```python
from build123d import *

# Parameters (mm, degrees)
PAD_DEPTH              = 6.05
SKETCH_W               = 3.6
SKETCH_H               = 14.9
POCKET_DEPTH           = 4.3
POCKET001_DEPTH        = 1.45
POCKET001_DEPTH_BACK   = 13.45
SKETCH004_W            = 0.55
SKETCH004_H            = 10
POCKET002_DEPTH        = 4.3
SKETCH005_W            = 1.2
SKETCH005_H            = 2.2
POCKET003_DEPTH        = 1.751
POCKET004_DEPTH        = 2.001
POCKET004_DEPTH_BACK   = 14.001
SKETCH007_W            = 0.5
SKETCH007_H            = 0.5
POCKET005_DEPTH        = 2.001
POCKET005_DEPTH_BACK   = 14.001
SKETCH008_W            = 0.2
SKETCH008_H            = 0.45
PAD001_DEPTH           = 4.85
LINEARPATTERN_COUNT    = 6
LINEARPATTERN_PITCH    = 2
POCKET006_DEPTH        = 12
SKETCH010_W            = 1.6
SKETCH010_H            = 0.2
POCKET007_DEPTH        = 2.951
POCKET007_DEPTH_BACK   = 1.751
LINEARPATTERN001_COUNT = 7
LINEARPATTERN001_PITCH = 2
SKETCH011_W            = 0.5
SKETCH011_H            = 0.5
POCKET008_DEPTH        = 0.001
POCKET008_DEPTH_BACK   = 6.051
LINEARPATTERN002_COUNT = 7
LINEARPATTERN002_PITCH = 2


with BuildPart() as part:
    # Sketch001 → Pad (new body)
    with BuildSketch(Plane.XY):
        with BuildLine():
            Line((-2.95, 1.5), (-2.95, -13.5))
            ThreePointArc((-2.95, -13.5), (-2.803553, -13.853553), (-2.45, -14))
            Line((-2.45, -14), (1.25, -14))
            ThreePointArc((1.25, -14), (1.603553, -13.853553), (1.75, -13.5))
            Line((1.75, -13.5), (1.75, 1.5))
            ThreePointArc((1.75, 1.5), (1.603553, 1.853553), (1.25, 2))
            Line((1.25, 2), (-2.45, 2))
            ThreePointArc((-2.45, 2), (-2.803553, 1.853553), (-2.95, 1.5))
        make_face()
    extrude(amount=PAD_DEPTH)

    # Sketch (on DatumPlane) → Pocket (cut)
    with BuildSketch(Plane.XY.offset(6.05)):
        with Locations((-0.6, -6)):
            Rectangle(SKETCH_W, SKETCH_H)
    extrude(amount=-POCKET_DEPTH, mode=Mode.SUBTRACT)

    # Sketch003 → Pocket001 (cut, two sides)
    with BuildSketch(Plane.XZ) as pocket001_sk:
        Polygon((1.5, 6.05), (1.2, 6.05), (1.2, 5.55), align=None)
        Polygon((-2.7, 6.05), (-2.4, 5.55), (-2.4, 6.05), align=None)
        Polygon((-2.4, 1.75), (-0.3, 1.75), (-0.9, 1.07), (-2.4, 1.07), align=None)
    extrude(amount=-POCKET001_DEPTH, mode=Mode.SUBTRACT)
    extrude(pocket001_sk.sketch, amount=POCKET001_DEPTH_BACK, mode=Mode.SUBTRACT)

    # Sketch004 (on DatumPlane) → Pocket002 (cut)
    with BuildSketch(Plane.XY.offset(6.05)):
        with Locations((1.475, -6)):
            Rectangle(SKETCH004_W, SKETCH004_H)
    extrude(amount=-POCKET002_DEPTH, mode=Mode.SUBTRACT)

    # Sketch005 → Pocket003 (cut, through all)
    with BuildSketch(Plane.YZ):
        with Locations((0.85, 2.93)):
            Rectangle(SKETCH005_W, SKETCH005_H)
        with Locations((-12.85, 2.93)):
            Rectangle(SKETCH005_W, SKETCH005_H)
    extrude(amount=POCKET003_DEPTH, mode=Mode.SUBTRACT)

    # Sketch006 → Pocket004 (cut, two sides)
    with BuildSketch(Plane.XZ) as pocket004_sk:
        with BuildLine():
            Line((0.45, 5.85), (0.45, 4.05))
            Line((0.45, 4.05), (-0.55, 4.05))
            Line((-0.55, 4.05), (-0.55, 5.85))
            ThreePointArc((-0.55, 5.85), (-0.608579, 5.991421), (-0.75, 6.05))
            Line((0.65, 6.05), (-0.75, 6.05))
            ThreePointArc((0.65, 6.05), (0.508579, 5.991421), (0.45, 5.85))
        make_face()
    extrude(amount=-POCKET004_DEPTH, mode=Mode.SUBTRACT)
    extrude(pocket004_sk.sketch, amount=POCKET004_DEPTH_BACK, mode=Mode.SUBTRACT)

    # Sketch007 → Pocket005 (cut, two sides)
    with BuildSketch(Plane.XZ) as pocket005_sk:
        with Locations((1.5, 0.95)):
            Rectangle(SKETCH007_W, SKETCH007_H)
    extrude(amount=-POCKET005_DEPTH, mode=Mode.SUBTRACT)
    extrude(pocket005_sk.sketch, amount=POCKET005_DEPTH_BACK, mode=Mode.SUBTRACT)

    # Sketch008 → Pad001 (join)
    with BuildSketch(Plane.XY):
        with Locations((-2.3, -1)):
            Rectangle(SKETCH008_W, SKETCH008_H)
    pad001 = extrude(amount=PAD001_DEPTH)

    # LinearPattern: Pad001 ×6
    with Locations(*[(0, -i * LINEARPATTERN_PITCH, 0) for i in range(1, LINEARPATTERN_COUNT)]):
        add(pad001)

    # Sketch009 → Pocket006 (cut)
    with BuildSketch(Plane.XZ):
        with BuildLine():
            Line((-2.4, 4.95), (-2.2, 4.95))
            Line((-2.2, 4.95), (-2.2, 4.65))
            ThreePointArc((-2.2, 4.65), (-2.258579, 4.791421), (-2.4, 4.85))
            Line((-2.4, 4.85), (-2.4, 4.95))
        make_face()
    extrude(amount=POCKET006_DEPTH, mode=Mode.SUBTRACT)

    # Sketch010 → Pocket007 (cut, two sides)
    with BuildSketch(Plane.YZ) as pocket007_sk:
        with Locations((0, 0.1)):
            Rectangle(SKETCH010_W, SKETCH010_H)
    pocket007 = extrude(amount=-POCKET007_DEPTH, mode=Mode.SUBTRACT) + extrude(pocket007_sk.sketch, amount=POCKET007_DEPTH_BACK, mode=Mode.SUBTRACT)

    # LinearPattern001: Pocket007 ×7
    with Locations(*[(0, -i * LINEARPATTERN001_PITCH, 0) for i in range(1, LINEARPATTERN001_COUNT)]):
        add(pocket007, mode=Mode.SUBTRACT)

    # Sketch011 → Pocket008 (cut, two sides)
    with BuildSketch(Plane.XY) as pocket008_sk:
        Rectangle(SKETCH011_W, SKETCH011_H)
    pocket008 = extrude(amount=-POCKET008_DEPTH, mode=Mode.SUBTRACT) + extrude(pocket008_sk.sketch, amount=POCKET008_DEPTH_BACK, mode=Mode.SUBTRACT)

    # LinearPattern002: Pocket008 ×7
    with Locations(*[(0, -i * LINEARPATTERN002_PITCH, 0) for i in range(1, LINEARPATTERN002_COUNT)]):
        add(pocket008, mode=Mode.SUBTRACT)


solid = part.part
```
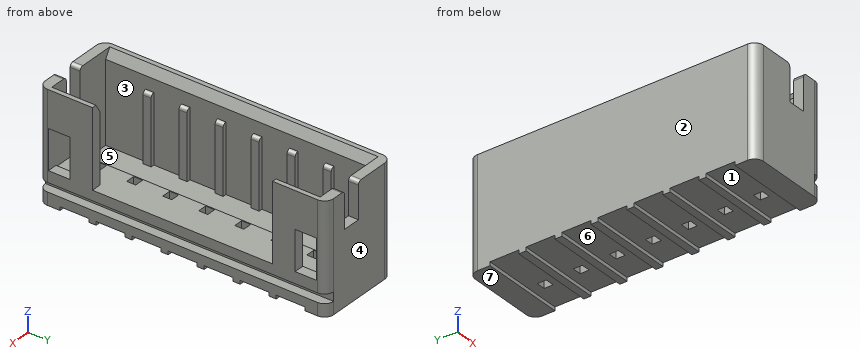
Geometry check sheet. Reference: the model listing, model coordinates, mm. Face numbers are marked on the shaded views. A direction names the side the tool comes from. Coordinates: 2 decimals unless noted, no trailing zeros. Order: outer loops, then holes, each group sorted by start corner. A loop starts at its lowest first (then second) coordinate and runs counter-clockwise, first axis right, second up. Notation, with made-up numbers: M -8,-36 L 7,-36 A23 cw 7,-10 Z; hole C -32.75,13 d1. An arc over 180 degrees is marked long. Answer as a JSON object with one key per item and string values.
Q1. Cross-section at B-B on y = -7. Record the cut outline in (x, z).
Results are:
{"outline": "M -2.95,0 L 1.75,0 L 1.75,0.7 L 1.25,0.7 L 1.25,1.2 L 1.75,1.2 L 1.75,1.75 L -0.3,1.75 L -0.9,1.07 L -2.2,1.07 L -2.2,4.65 A0.2 ccw -2.4,4.85 L -2.4,5.55 L -2.7,6.05 L -2.95,6.05 Z"}
Q2. Cross-section at A-A on y = 1. Record the cut outline in (x, z), and give its area (3 significant figures).
Results are:
{"outline": "M -2.95,0 L 1.75,0 L 1.75,0.7 L 1.25,0.7 L 1.25,1.2 L 1.75,1.2 L 1.75,1.83 L 1.2,1.83 L 1.2,1.75 L -0.3,1.75 L -0.9,1.07 L -2.4,1.07 L -2.4,5.55 L -2.7,6.05 L -2.95,6.05 Z; M 1.2,4.03 L 1.75,4.03 L 1.75,6.05 L 1.5,6.05 L 1.2,5.55 Z", "area": "10.1 mm²"}
Q3. Tool access check on the marked faces 5, 6 and 7. Record the directions out of +Z, -Z, +X, -X, +Y, -Y that give a thin tool (end or side, any length) a straight path to the whole face; none if there is none.
Results are:
{"face 5": "+Z", "face 6": "-Z, +X, -X", "face 7": "-Z, +X, -X, +Y, -Y"}
Q4. Cross-section at C-C on z = 3.25. Give the number of separate pieces and of enclosed holes in the cut face, and give its area (3 significant figures).
Results are:
{"separate pieces": "3", "enclosed holes": "0", "area": "15.1 mm²"}
Q5. Depth check by flat-ended pin: pin 1 Ø1.5 at (x, y) = (-2, -6.5) entering from -Z. Enter the tip coordinate at first touch or a pass-through.
Results are:
{"pin 1": "stops at z = 0"}
Q6. Scan lines: line 1 (Y direction, x = -1.1, z = 3.75); line 2 (X direction, y = -13, z = 5); line 3 (X direction, y = -13, z = 0.75). Record each from-to range of solid material in increasing order.
Results are:
{"line 1": "y = -14 to -13.45, 1.45 to 2", "line 2": "x = -2.95 to -2.4, 1.2 to 1.75", "line 3": "x = -2.95 to 1.25"}
Q7. Release check for a two-part mould opening along Y. For the marked faces 1, 2, 3 and 4 record: released by +Y, released by -Y, zero draft, split by the parting line, or undercut.
Results are:
{"face 1": "undercut", "face 2": "zero draft", "face 3": "undercut", "face 4": "released by +Y"}
